Geometry check sheet. Reference: drawing and pictorial views, mm from the part's lowest x, y, z. Coordinates: 2 decimals unless noted, no trailing zeros. Loops run counter-clockwise (first coordinate to the right, second up) from the corner with the lowest first, then second, coordinate; pieces in that order, holes last. Notation, with made-up numbers: (14.25, 81.5) -> (61.25, 81.5) arc R12 cw to (61.25, 95.5) -> close; hole circle Ø7 at (67, 86). An arc over 180 degrees is marked (long way). Answer as a JSON object with one key per item and string values.
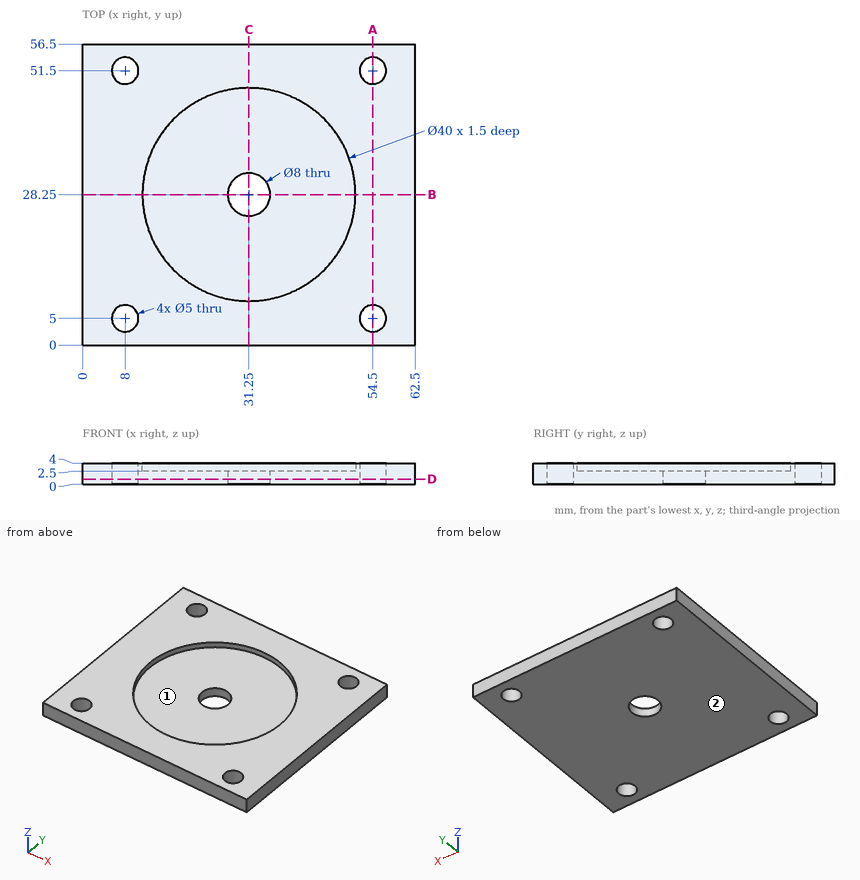
1. Thickness scan on probe 1 along Y at (x, z) = (54.5, 0.9); probe 2 along Y at (x, z) = (31.25, 2.9); probe 3 along Y at (x, z) = (7.5, 2.8). Record the ranges inside material, lowest first. Write a range as from..to.
Evaluation:
{"probe 1": "y = 0..2.5, 7.5..49, 54..56.5", "probe 2": "y = 0..8.25, 48.25..56.5", "probe 3": "y = 0..2.55, 7.45..49.05, 53.95..56.5"}
2. Mould release check, pull along Y, two halves, no side actions. Record for the marked faces 1 and 2: released by +Y, released by -Y, zero draft, split by the parting line, or undercut.
Evaluation:
{"face 1": "undercut", "face 2": "zero draft"}
3. Depth check by flat-ended pin: P1, Ø4.5, axis at x = 8, y = 51.5, coming from the +Z side; P2, Ø9, axis at x = 31.25, y = 28.25, coming from the +Z side. Enter the tip coordinate at first touch or a pass-through.
Evaluation:
{"P1": "passes through", "P2": "stops at z = 2.5"}
4. Section check B-B, the plane y = 28.25. Record the boundary of the cut face in (x, z), then the cut area to 3 significant figures.
Evaluation:
{"outline": "(0, 0) -> (27.25, 0) -> (27.25, 2.5) -> (11.25, 2.5) -> (11.25, 4) -> (0, 4) -> close; (35.25, 0) -> (62.5, 0) -> (62.5, 4) -> (51.25, 4) -> (51.25, 2.5) -> (35.25, 2.5) -> close", "area": "170 mm^2"}
5. Section check D-D, the plane z = 1. Record the boundary of the cut face in (x, y).
Evaluation:
{"outline": "(0, 0) -> (62.5, 0) -> (62.5, 56.5) -> (0, 56.5) -> close; hole circle Ø5 at (8, 5); hole circle Ø5 at (8, 51.5); hole circle Ø8 at (31.25, 28.25); hole circle Ø5 at (54.5, 5); hole circle Ø5 at (54.5, 51.5)"}
6. Section check C-C, the plane x = 31.25. Record the boundary of the cut face in (y, z).
Evaluation:
{"outline": "(0, 0) -> (24.25, 0) -> (24.25, 2.5) -> (8.25, 2.5) -> (8.25, 4) -> (0, 4) -> close; (32.25, 0) -> (56.5, 0) -> (56.5, 4) -> (48.25, 4) -> (48.25, 2.5) -> (32.25, 2.5) -> close"}
7. Section check A-A, the plane x = 54.5. Record the boundary of the cut face in (y, z), then the cut area to 3 significant figures.
Evaluation:
{"outline": "(0, 0) -> (2.5, 0) -> (2.5, 4) -> (0, 4) -> close; (7.5, 0) -> (49, 0) -> (49, 4) -> (7.5, 4) -> close; (54, 0) -> (56.5, 0) -> (56.5, 4) -> (54, 4) -> close", "area": "186 mm^2"}
